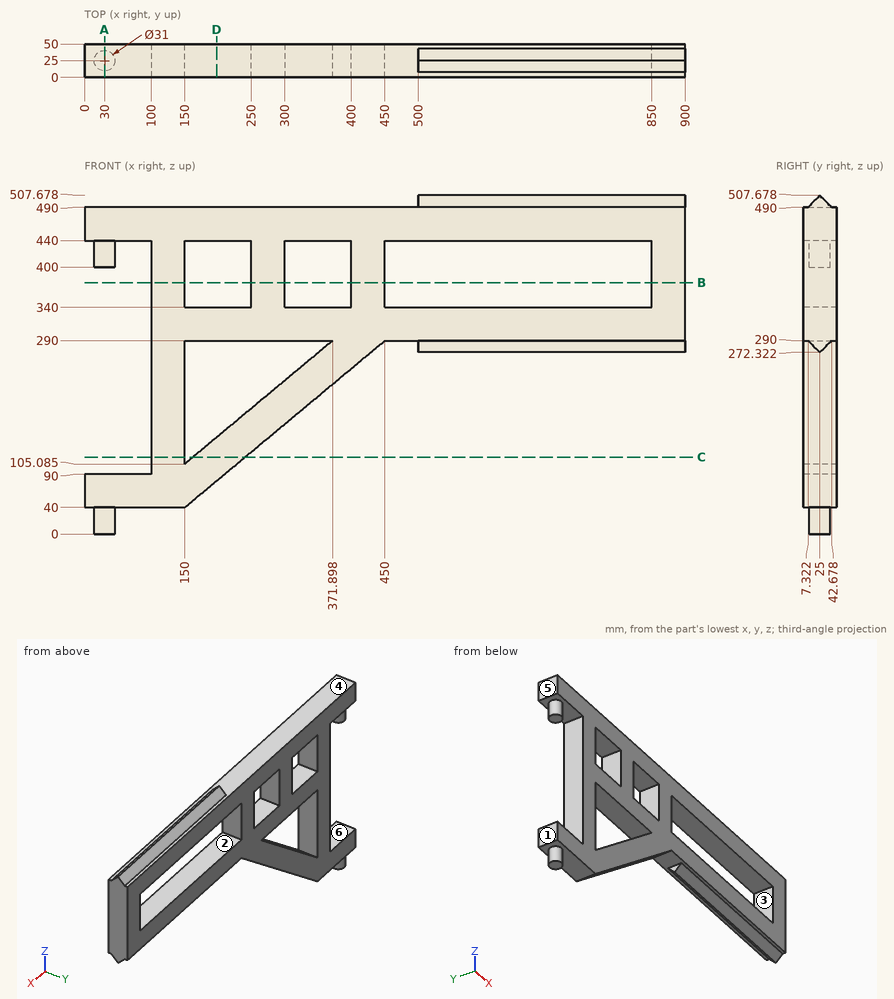
Job drawing, mm, ordinate dimensions from the low corner. One solid piece. A direction names the side the tool comes from. Coordinates: 2 decimals unless noted, no trailing zeros. Order: outer loops, then holes, each group sorted by start corner. A loop starts at its lowest first (then second) coordinate and runs counter-clockwise, first axis right, second up. Notation, with made-up numbers: (3, -8.75) -> (36, -8.75) arc R6 ccw to (36, -4.75) -> close; hole circle Ø3 at (-37.5, 16). An arc over 180 degrees is marked (long way). Answer in a Markdown table with one row per item. Add a question column.
Q1. Which spindle directions (+Z, -Z, +X, -X, +Y, -Y) get a long thin tool onto all of the face, cutting with end or side? Do the marked faces 1 and 2. Say none if no direction does.
Q2. Band-saw the part on C-C, the plane z = 115.5. List the corners of the cut face in (x, y).
Q3. Mould opens along Z. For the marked faces 3, 4, 5 and 6 say: +Z half, -Z half, draft (parallel to the pull), parting line (faces both ways), or undercut.
Q4. Band-saw the part on A-A, the plane x = 30. List the corners of the cut face in (y, z).
Q5. Wall check: line 1 along X through (y, z) = (8.5, 403.5); line 2 along Z through (x, y) = (41.5, 14); line 3 along Z through (x, y) = (619.5, 3.5). Give the ranges that are in metal, low to high. Write a range as [from, to].
Q6. Band-saw the part on B-B, the plane z = 377. List the corners of the cut face in (x, y), then the cut area to 3 significant figures.
Q7. Drop flat-ended pins along their axis: pin 1 (2 mm diameter, centred on y = 23.5, z = 212, fed in from +X); pin 2 (8 mm diameter, centred on x = 284.5, y = 12.5, fed in from -Z); pin 3 (25 mm diameter, centred on y = 22, z = 278.5, fed in from -X); pin 4 (15 mm diameter, centred on x = 43.5, y = 13.5, fed in from -Z). Give the stop position or say it passes through.
Q8. Band-saw the part on D-D, the plane x = 198. List the corners of the cut face in (y, z) (1 decimal).
Answers follow:
| question | item | result |
|---|---|---|
| 1 | face 1 | +Z, -Z, -X, +Y, -Y |
| 1 | face 2 | +Y, -Y |
| 2 | outline | (100, 0) -> (150, 0) -> (150, 50) -> (100, 50) -> close; (162.5, 0) -> (240.6, 0) -> (240.6, 50) -> (162.5, 50) -> close |
| 3 | face 3 | undercut |
| 3 | face 4 | +Z half |
| 3 | face 5 | draft |
| 3 | face 6 | undercut |
| 4 | outline | (0, 40) -> (9.5, 40) -> (9.5, 0) -> (40.5, 0) -> (40.5, 40) -> (50, 40) -> (50, 90) -> (0, 90) -> close; (0, 440) -> (9.5, 440) -> (9.5, 400) -> (40.5, 400) -> (40.5, 440) -> (50, 440) -> (50, 490) -> (0, 490) -> close |
| 5 | line 1 | [100, 150], [250, 300], [400, 450], [850, 900] |
| 5 | line 2 | [40, 90], [440, 490] |
| 5 | line 3 | [290, 340], [440, 490] |
| 6 | outline | (100, 0) -> (150, 0) -> (150, 50) -> (100, 50) -> close; (250, 0) -> (300, 0) -> (300, 50) -> (250, 50) -> close; (400, 0) -> (450, 0) -> (450, 50) -> (400, 50) -> close; (850, 0) -> (900, 0) -> (900, 50) -> (850, 50) -> close |
| 6 | area | 10,000 mm^2 |
| 7 | pin 1 | x = 357.6 |
| 7 | pin 2 | z = 148.75 |
| 7 | pin 3 | x = 100 |
| 7 | pin 4 | z = 0 |
| 8 | outline | (0, 80) -> (50, 80) -> (50, 145.1) -> (0, 145.1) -> close; (0, 290) -> (50, 290) -> (50, 340) -> (0, 340) -> close; (0, 440) -> (50, 440) -> (50, 490) -> (0, 490) -> close |
